Source: three-view drawing plus pictorial views. Frame: mm from the lowest corner of the part. A direction names the side the tool comes from. Round coordinates to 2 decimals unless told otherwise and drop trailing zeros. Loops run counter-clockwise (first coordinate to the right, second up) from the corner with the lowest first, then second, coordinate; pieces in that order, holes last. Notation, with made-up numbers: M 44.25,36 L 57.25,36 A29 cw 57.25,70 Z; hole C 4.25,77 d2. An arc over 180 degrees is marked long. Return JSON: item names as keys, results as strings. Group by question number.
1) Contact query for flat-ended pins moving along their axis: P1, Ø20, axis at x = 67.5, y = 33, coming from the +Z side; P2, Ø6, axis at y = 34, z = 7, coming from the +X side; P3, Ø6, axis at x = 11.5, z = 6, coming from the -Y side; P4, Ø12, axis at x = 47, z = 45.5, coming from the -Y side. Output: stop coordinate, or through.
2) Section C-C (x = 58). Output: boundary loops of the cut face in (y, z).
3) Section B-B (y = 7). Output: boundary loops of the cut face in (x, z), plus the area to 3 significant figures.
4) Section D-D (x = 25). Output: boundary loops of the cut face in (y, z).
5) Material intervals for line 1 (X direction, y = 38.5, z = 27.5); line 2 (X direction, y = 43.5, z = 14); line 3 (Z direction, x = 86.5, y = 27.5), sorted ascending. Write a range as from..to.
6) Section A-A (z = 23.5). Output: boundary loops of the cut face in (x, y).
7) Access query for the marked faces 1, 2, 3 and 4. Directions: +Z, -Z, +X, -X, +Y, -Y. A direction counts if a zero-diameter tool reaches every point of the face in a straight line with its end or side. Return the directions, or none.
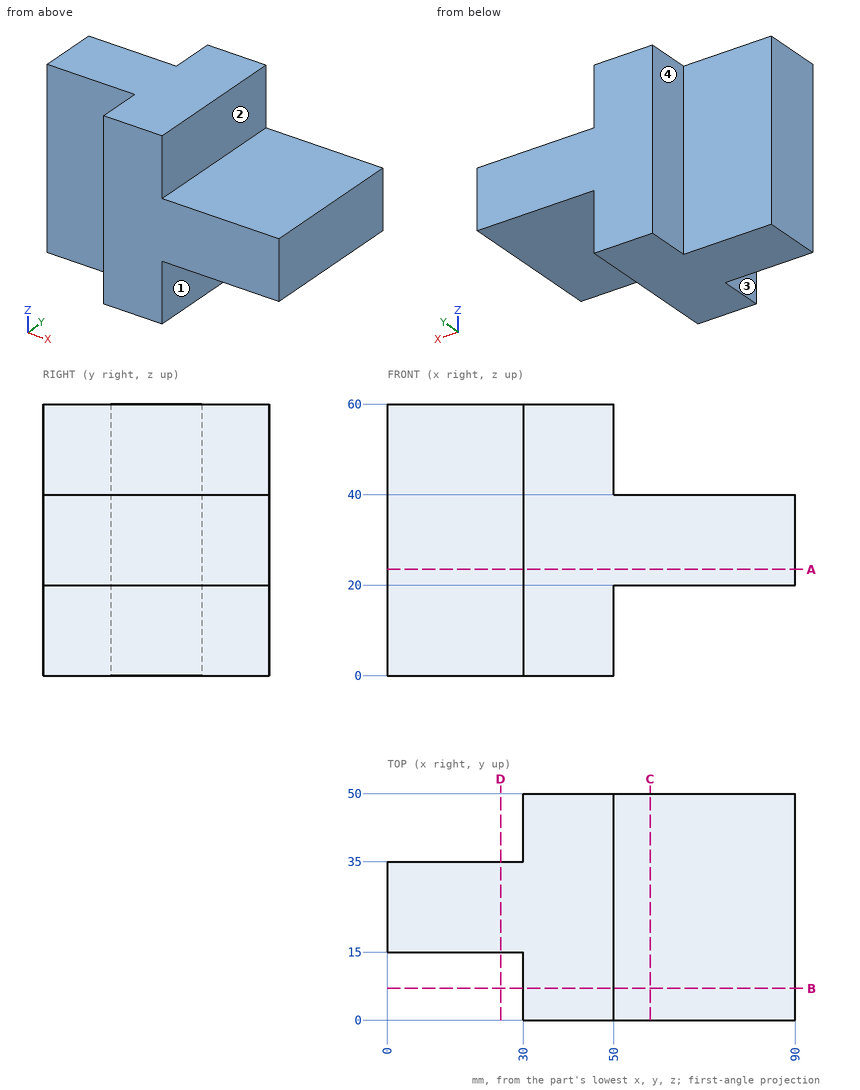
Returned:
{
 "1": {"P1": "stops at z = 40", "P2": "stops at x = 50", "P3": "stops at y = 15", "P4": "stops at y = 0"},
 "2": {"outline": "M 0,20 L 50,20 L 50,40 L 0,40 Z"},
 "3": {"outline": "M 30,0 L 50,0 L 50,20 L 90,20 L 90,40 L 50,40 L 50,60 L 30,60 Z", "area": "2,000 mm^2"},
 "4": {"outline": "M 15,0 L 35,0 L 35,60 L 15,60 Z"},
 "5": {"line 1": "x = 30..90", "line 2": "x = 30..50", "line 3": "z = 20..40"},
 "6": {"outline": "M 0,15 L 30,15 L 30,0 L 90,0 L 90,50 L 30,50 L 30,35 L 0,35 Z"},
 "7": {"face 1": "-Z, +X, +Y, -Y", "face 2": "+Z, +X, +Y, -Y", "face 3": "+Z, -Z, -X, -Y", "face 4": "+Z, -Z, -X, +Y"}
}
